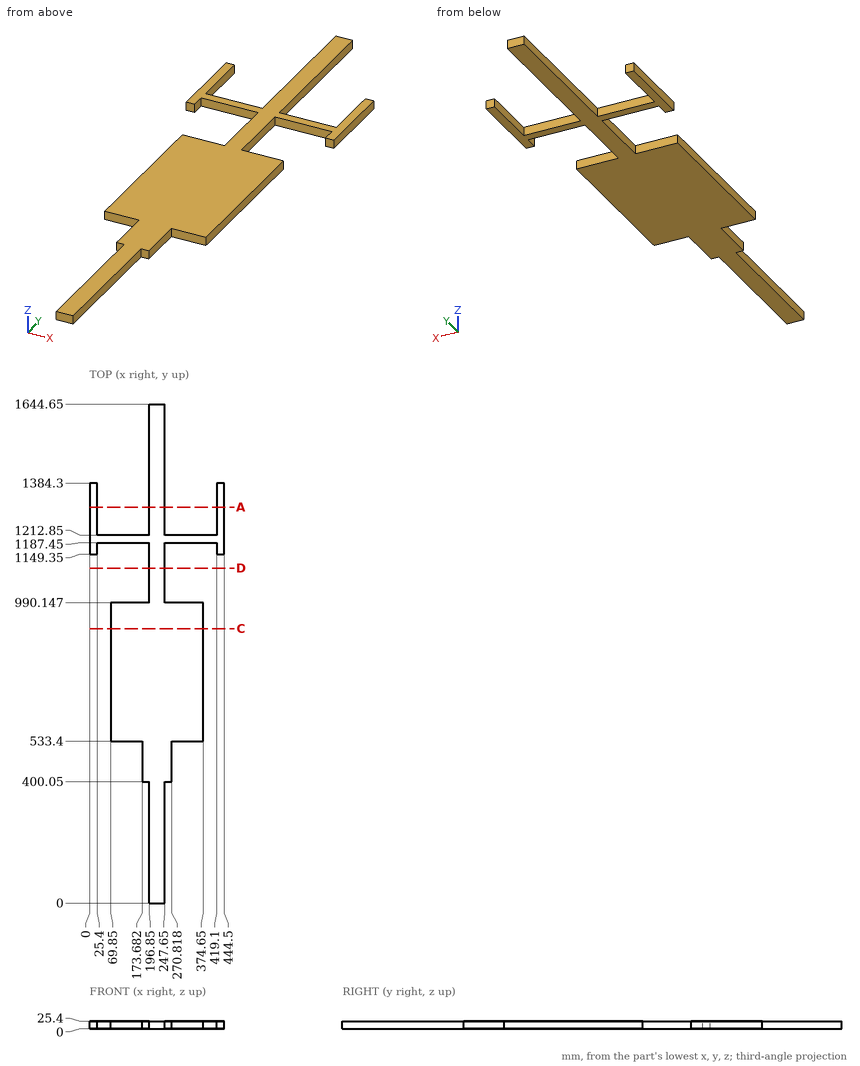
Drawing for the job (mm, zero at the part's lowest x, y, z). Give positions to 0.01 mm unless a question says otherwise; leave off trailing zeros. Order: outer loops, then holes, each group sorted by start corner. A loop starts at its lowest first (then second) coordinate and runs counter-clockwise, first axis right, second up. Notation, with made-up numbers: M 53,-35.75 L 99,-35.75 A19 cw 99,-15.75 Z; hole C 10.5,8 d6. An arc over 180 degrees is marked long. Put each result on its own line as item: value. Start each with the question number.
(1) Saw through at A-A, the plane y = 1304.5. Write the cut outline in (x, z).
(2) Saw through at C-C, the plane y = 904.5. Write the cut outline in (x, z), then the cut area to 3 significant figures.
(3) Drill centre lines: line 1 along X through (y, z) = (1238, 21.5); line 2 along Y through (x, z) = (155, 19); line 3 along Y through (x, z) = (187, 22.5). Where is each one in solid material? Low to high.
(4) Flat gauge pins, fed straight in: pin 1 Ø12 at (y, z) = (1032.5, 3) entering from +X; pin 2 Ø12.5 at (x, z) = (9, 13) entering from +Y; pin 3 Ø7.5 at (y, z) = (667.5, 19) entering from -X; pin 4 Ø1.5 at (y, z) = (1349.5, 14.5) entering from -X. Where does each tip first touch, or does it go through?
(5) Saw through at D-D, the plane y = 1103.5. Write the cut outline in (x, z), then the cut area to 3 significant figures.
Check result:
1. outline: M 0,0 L 25.4,0 L 25.4,25.4 L 0,25.4 Z; M 196.85,0 L 247.65,0 L 247.65,25.4 L 196.85,25.4 Z; M 419.1,0 L 444.5,0 L 444.5,25.4 L 419.1,25.4 Z
2. outline: M 69.85,0 L 374.65,0 L 374.65,25.4 L 69.85,25.4 Z
2. area: 7,740 mm2
3. line 1: x = 0 to 25.4, 196.85 to 247.65, 419.1 to 444.5
3. line 2: y = 533.4 to 990.15, 1187.45 to 1212.85
3. line 3: y = 400.05 to 990.15, 1187.45 to 1212.85
4. pin 1: stops at x = 247.65
4. pin 2: stops at y = 1384.3
4. pin 3: stops at x = 69.85
4. pin 4: stops at x = 0
5. outline: M 196.85,0 L 247.65,0 L 247.65,25.4 L 196.85,25.4 Z
5. area: 1,290 mm2
